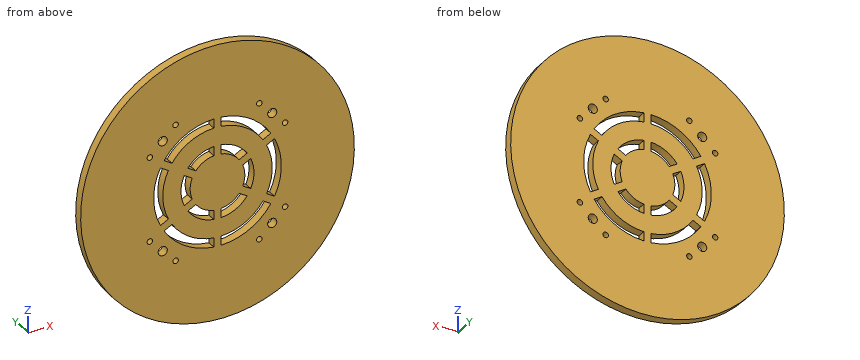
from build123d import *

# Parameters (mm, degrees)
SKETCH1_R           = 75
BOSS_EXTRUDE1_DEPTH = 5
SKETCH2_R           = 2.5
SKETCH2_R_2         = 1.5
CUT_EXTRUDE1_DEPTH  = 5
SKETCH3_R           = 35
SKETCH3_R_2         = 30
SKETCH3_R_3         = 20
SKETCH3_R_4         = 15
CUT_EXTRUDE3_DEPTH  = 5
SKETCH4_W           = 4
SKETCH4_H           = 72.786785362
BOSS_EXTRUDE2_DEPTH = 5
CIRPATTERN1_COUNT   = 6


with BuildPart() as part:
    # Sketch1 → Boss-Extrude1 (new body)
    with BuildSketch(Plane(origin=(0, 0, 0), x_dir=(1, 0, 0), z_dir=(0, 1, 0))):
        with Locations(Location((0, 0, 0), (0, 0, 270))):
            Circle(SKETCH1_R)
    extrude(amount=BOSS_EXTRUDE1_DEPTH)

    # Sketch2 → Cut-Extrude1 (cut)
    with BuildSketch(Plane(origin=(0, 5, 0), x_dir=(1, 0, 0), z_dir=(0, 1, 0))):
        with Locations(Location((-29.999005192, 29.999005192, 0), (0, 0, 270))):
            Circle(SKETCH2_R)
        with Locations(Location((29.999005192, 29.999005192, 0), (0, 0, 270))):
            Circle(SKETCH2_R)
        with Locations(Location((29.999005192, -29.999005192, 0), (0, 0, 270))):
            Circle(SKETCH2_R)
        with Locations(Location((-29.999005192, -29.999005192, 0), (0, 0, 270))):
            Circle(SKETCH2_R)
        with Locations(Location((-22.92793738, 37.070073004, 0), (0, 0, 270))):
            Circle(SKETCH2_R_2)
        with Locations(Location((-37.070073004, 22.92793738, 0), (0, 0, 270))):
            Circle(SKETCH2_R_2)
        with Locations(Location((22.92793738, 37.070073004, 0), (0, 0, 270))):
            Circle(SKETCH2_R_2)
        with Locations(Location((37.070073004, 22.92793738, 0), (0, 0, 270))):
            Circle(SKETCH2_R_2)
        with Locations(Location((-37.070073004, -22.92793738, 0), (0, 0, 270))):
            Circle(SKETCH2_R_2)
        with Locations(Location((-22.92793738, -37.070073004, 0), (0, 0, 270))):
            Circle(SKETCH2_R_2)
        with Locations(Location((22.92793738, -37.070073004, 0), (0, 0, 270))):
            Circle(SKETCH2_R_2)
        with Locations(Location((37.070073004, -22.92793738, 0), (0, 0, 270))):
            Circle(SKETCH2_R_2)
    extrude(amount=-CUT_EXTRUDE1_DEPTH, mode=Mode.SUBTRACT)

    # Sketch3 → Cut-Extrude3 (cut)
    # profile 1 of 2: a face of its own
    with BuildSketch(Plane(origin=(0, 5, 0), x_dir=(1, 0, 0), z_dir=(0, 1, 0))):
        with Locations(Location((0, 0, 0), (0, 0, 270))):
            Circle(SKETCH3_R)
        with Locations(Location((0, 0, 0), (0, 0, 270))):
            Circle(SKETCH3_R_2, mode=Mode.SUBTRACT)
    # profile 2 of 2: a face of its own
    with BuildSketch(Plane(origin=(0, 5, 0), x_dir=(1, 0, 0), z_dir=(0, 1, 0))):
        with Locations(Location((0, 0, 0), (0, 0, 270))):
            Circle(SKETCH3_R_3)
        with Locations(Location((0, 0, 0), (0, 0, 270))):
            Circle(SKETCH3_R_4, mode=Mode.SUBTRACT)
    extrude(amount=-CUT_EXTRUDE3_DEPTH, mode=Mode.SUBTRACT)


with BuildPart() as cut_extrude3_piece_1:
    # of the separate pieces the step leaves, piece 1, a body of its own (cut_extrude3_pieces)
    add(part.part.solids().sort_by_distance((0, 0, 75))[0])



with BuildPart() as cut_extrude3_piece_2:
    # of the separate pieces the step leaves, piece 2, a body of its own (cut_extrude3_pieces)
    add(part.part.solids().sort_by_distance((0, 0, 30))[0])


with BuildPart() as cut_extrude3_piece_3:
    # of the separate pieces the step leaves, piece 3, a body of its own (cut_extrude3_pieces)
    add(part.part.solids().sort_by_distance((0, 0, 15))[0])


with BuildPart() as cut_extrude3_piece_1_1:
    add(cut_extrude3_piece_1.part)

    add(cut_extrude3_piece_2.part)  # Boss-Extrude2 merges Cut-Extrude3 piece 2

    add(cut_extrude3_piece_3.part)  # Boss-Extrude2 merges Cut-Extrude3 piece 3
    # Sketch4 → Boss-Extrude2 (add)
    with BuildSketch(Plane(origin=(0, 5, 0), x_dir=(1, 0, 0), z_dir=(0, 1, 0))):
        Rectangle(SKETCH4_W, SKETCH4_H)
    boss_extrude2 = extrude(amount=-BOSS_EXTRUDE2_DEPTH)

    # CirPattern1: Boss-Extrude2 ×6 about axis
    cirpattern1_axis = Axis((0, 0, 0), (0, 1, 0))
    for i in range(1, CIRPATTERN1_COUNT):
        add(boss_extrude2.rotate(cirpattern1_axis, i * 360 / CIRPATTERN1_COUNT))


solid = cut_extrude3_piece_1_1.part
Read the model definition and answer for the solid it produces. Units are mm, in the model's axes. Round coordinates to 2 decimals unless told otherwise and drop trailing zeros. Order: outer loops, then holes, each group sorted by start corner. A loop starts at its lowest first (then second) coordinate and runs counter-clockwise, first axis right, second up.
1) Flat-ended cylindrical pins translate along their axes: pin 1 (4 mm diameter, centred on x = 30, z = 30, fed in from -Y); pin 2 (1.5 mm diameter, centred on y = 2.5, z = -17, fed in from +X); pin 3 (5 mm diameter, centred on x = -22.93, z = 37.07, fed in from -Y); pin 4 (2.5 mm diameter, centred on y = 3, z = 17, fed in from -X). Find the tip coordinate at first contact, or state that the pin passes through.
2) The part is cut by section A-A on z = 0. Write down the section's boundary in (x, y), plus the area to 3 significant figures.
3) Straight lines are drawn through the part: L1, parallel to X at y = 1.45, z = -0.5; L2, parallel to X at y = 0.55, z = -13.5 (3 decimals); L3, parallel to Z at x = 22, y = 2.25. For each, find the intervals that lie inside material, in ascending order.
4) The part is cut by section C-C on y = 1.3. Give the number of separate pieces and of enclosed holes in the cut face, plus the area to 3 significant figures.
5) The part is cut by section D-D on x = -59. Write down the section's boundary in (y, z).
6) The part is cut by section B-B on x = 51. Write down the section's boundary in (y, z).
Resolved:
1. pin 1: passes through
1. pin 2: stops at x = 73.22
1. pin 3: stops at y = 0
1. pin 4: stops at x = -73.33
2. outline: (-75, 0) - (-35, 0) - (-35, 5) - (-75, 5) - close; (-30, 0) - (-20, 0) - (-20, 5) - (-30, 5) - close; (-15, 0) - (15, 0) - (15, 5) - (-15, 5) - close; (20, 0) - (30, 0) - (30, 5) - (20, 5) - close; (35, 0) - (75, 0) - (75, 5) - (35, 5) - close
2. area: 650 mm2
3. L1: x = -75 to -35, -30 to -19.99, -14.99 to 14.99, 19.99 to 30, 35 to 75
3. L2: x = -73.775 to -32.292, -27.383 to -14.756, -6.538 to 6.538, 14.756 to 27.383, 32.292 to 73.775
3. L3: z = -71.7 to -38.25, -35.89 to -27.22, -20.4 to 20.4, 27.22 to 35.89, 38.25 to 71.7
4. separate pieces: 1
4. enclosed holes: 24
4. area: 16,200 mm2
5. outline: (0, -46.3) - (5, -46.3) - (5, 46.3) - (0, 46.3) - close
6. outline: (0, -54.99) - (5, -54.99) - (5, 54.99) - (0, 54.99) - close
